from build123d import *

# Parameters (mm, degrees)
RESSALTO_EXTRUS_O1_DEPTH = 18
ESBO_O2_R                = 1.5
CORTE_EXTRUS_O1_DEPTH    = 17


with BuildPart() as part:
    # Esboço1 → Ressalto-extrusão1 (new body)
    with BuildSketch(Plane.XY):
        with BuildLine():
            Line((10.087087811, 2), (15.8, 2))
            Line((15.8, 2), (15.8, 0))
            Line((15.8, 0), (7.8, 0))
            ThreePointArc((7.8, 0), (0.8, 7), (-6.2, 0))
            Line((-6.2, 0), (-14.2, 0))
            Line((-14.2, 0), (-14.2, 2))
            Line((-14.2, 2), (-8.487087811, 2))
            ThreePointArc((-8.487087811, 2), (0.8, 9.5), (10.087087811, 2))
        make_face()
    extrude(amount=RESSALTO_EXTRUS_O1_DEPTH)

    # Esboço2 → Corte-extrusão1 (cut)
    with BuildSketch(Plane(origin=(0, 2, 0), x_dir=(1, 0, 0), z_dir=(0, 1, 0))):
        with Locations((12.8, -9)):
            Circle(ESBO_O2_R)
        with Locations((-11.2, -9)):
            Circle(ESBO_O2_R)
    extrude(amount=-CORTE_EXTRUS_O1_DEPTH, mode=Mode.SUBTRACT)


solid = part.part
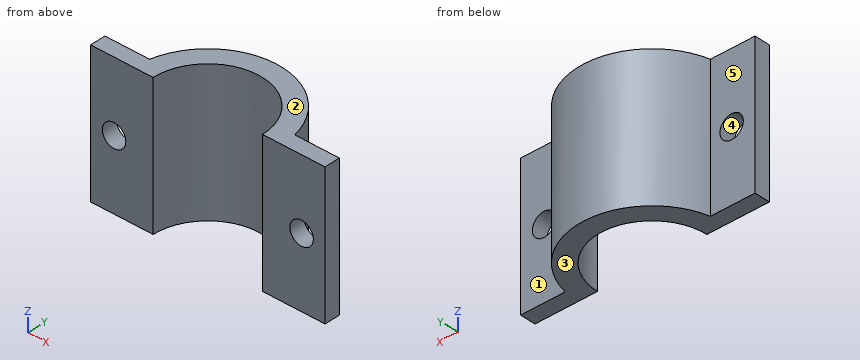
Read the model definition and answer for the solid it produces. Units are mm, in the model's axes. Face numbers are marked on the shaded views. A direction names the side the tool comes from. Coordinates: 2 decimals unless noted, no trailing zeros. Loops run counter-clockwise (first coordinate to the right, second up) from the corner with the lowest first, then second, coordinate; pieces in that order, holes last.
Q1. The part is cut by section A-A on y = 1.5. Write down the section's boundary in (x, z).
Q2. Consider probe 1 along Z at (x, y) = (12.8, 1.3); probe 2 along X at (y, z) = (1.5, 8); probe 3 along X at (y, z) = (1.25, 9). Determine where each line is inside the solid, lowest interval first.
Q3. The mould has two halves that part along Z. Classify the marked faces 3, 4 and 5: +Z half, -Z half, draft (parallel to the pull), parting line (faces both ways), or undercut.
Q4. Each of these flat-tipped pins is pushed along its axis until it touches: pin 1 Ø1.5 at (x, z) = (-11, 9) entering from -Y; pin 2 Ø2 at (y, z) = (3.5, 12.5) entering from -X; pin 3 Ø4.5 at (x, z) = (14, 9) entering from +Y; pin 4 Ø10 at (x, z) = (6.5, 11.5) entering from +Y. Where does it stop, or does it pass through?
Q5. Which of the six approach directions +Z, -Z, +X, -X, +Y, -Y give full straight-line access (tool end or side, diameter ignored) to the marked faces 1 and 2?
Q6. The part is cut by section D-D on y = 4.75. Write down the section's boundary in (x, z), and give its area (3 significant figures).
Q7. The part is cut by section B-B on x = -11.2. Write down the section's boundary in (y, z), and give its area (3 significant figures).
Q8. The part is cut by section C-C on z = 9. Write down the section's boundary in (x, y).
Results below:
1. outline: (-14.2, 0) - (-6.04, 0) - (-6.04, 18) - (-14.2, 18) - close; (7.64, 0) - (15.8, 0) - (15.8, 18) - (7.64, 18) - close; hole circle Ø3 at (-11.2, 9); hole circle Ø3 at (12.8, 9)
2. probe 1: z = 0 to 7.5, 10.5 to 18
2. probe 2: x = -14.2 to -12.32, -10.08 to -6.04, 7.64 to 11.68, 13.92 to 15.8
2. probe 3: x = -14.2 to -12.7, -9.7 to -6.09, 7.69 to 11.3, 14.3 to 15.8
3. face 3: -Z half
3. face 4: undercut
3. face 5: draft
4. pin 1: passes through
4. pin 2: stops at x = -8.37
4. pin 3: stops at y = 2
4. pin 4: stops at y = 9.47
5. face 1: +Z, -Z, +X, +Y
5. face 2: +Z, +X, -X, +Y, -Y
6. outline: (-7.43, 0) - (-4.34, 0) - (-4.34, 18) - (-7.43, 18) - close; (5.94, 0) - (9.03, 0) - (9.03, 18) - (5.94, 18) - close
6. area: 111 mm2
7. outline: (0, 0) - (2, 0) - (2, 7.5) - (0, 7.5) - close; (0, 10.5) - (2, 10.5) - (2, 18) - (0, 18) - close
7. area: 30.0 mm2
8. outline: (-14.2, 0) - (-12.7, 0) - (-12.7, 2) - (-14.2, 2) - close; (-9.7, 0) - (-6.2, 0) arc R7 cw to (7.8, 0) - (11.3, 0) - (11.3, 2) - (10.09, 2) arc R9.5 ccw to (-8.49, 2) - (-9.7, 2) - close; (14.3, 0) - (15.8, 0) - (15.8, 2) - (14.3, 2) - close
